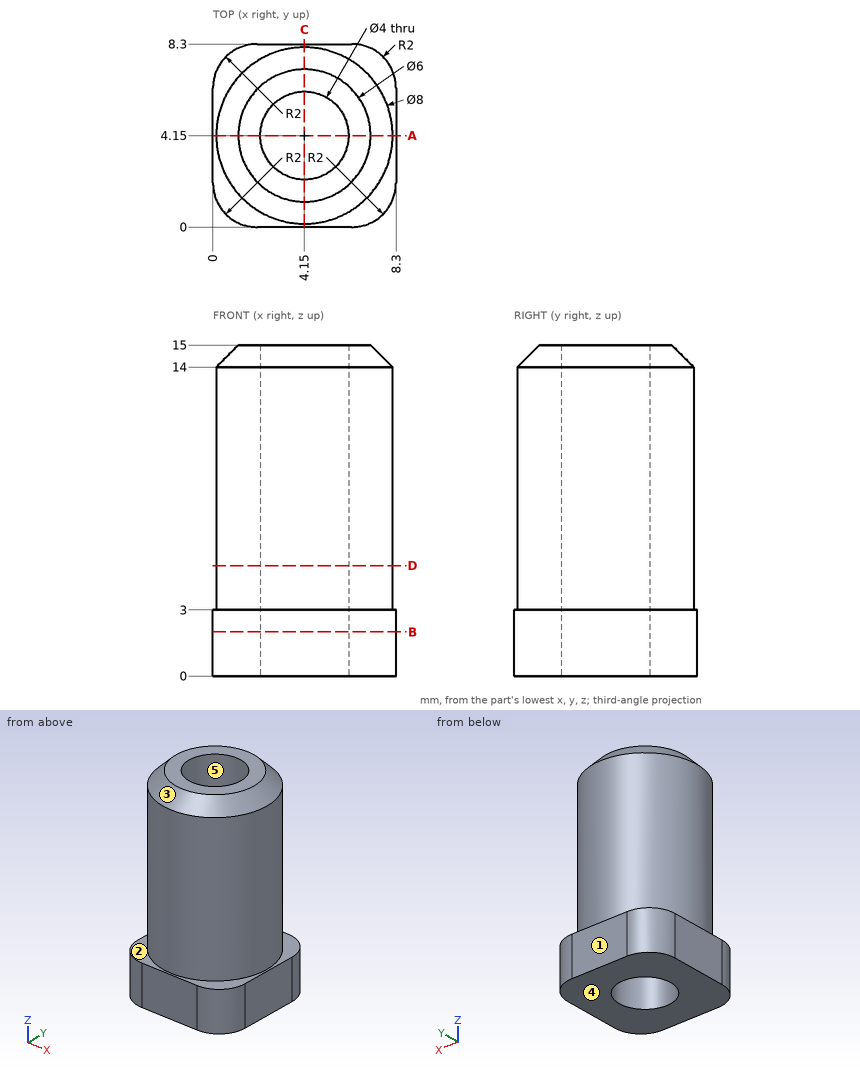
Could you check a few things on this drawing? It's one solid part, dimensions in mm from its lowest x, y, z. A direction names the side the tool comes from. Give positions to 0.01 mm unless a question says otherwise; leave off trailing zeros. Order: outer loops, then holes, each group sorted by start corner. A loop starts at its lowest first (then second) coordinate and runs counter-clockwise, first axis right, second up. Notation, with made-up numbers: (-13.75, 85.25) - (7.25, 85.25) arc R29 cw to (7.25, 113.25) - close; hole circle Ø10 at (5, 39.25). An arc over 180 degrees is marked (long way). Answer as a JSON object with one key per item and string values. Group by question number.
Item 1: For P1, Ø1.5, axis at x = 6.5, z = 11, coming from the +Y side, with a flat end and sliding along its axis, tell me the tip position at first contact or that it passes through.
Item 2: If we section it at D-D on z = 5: Please give me the cut outline in (x, y).
Item 3: If we mould it in two halves opening along X, with no side actions, what happens to the marked faces 3, 4 and 5? For each: pulls with the +X half, pulls with the -X half, needs draft (parallel to the pull), parting line crosses it, or undercut.
Item 4: If we section it at A-A on y = 4.15: Please give me the cut outline in (x, z).
Item 5: Please list where these lines run through material, in increasing order: probe 1 along Y at (x, z) = (4.15, 5); probe 2 along X at (y, z) = (4, 7.25); probe 3 along X at (y, z) = (4.75, 1.75).
Item 6: Which directions (+Z, -Z, +X, -X, +Y, -Y) give clear straight access to the entire face, cutting with the end or side of a thin tool? Please do the marked faces 1 and 2.
Item 7: If we section it at B-B on z = 2: Please give me the cut outline in (x, y), and give its area (3 significant figures).
Result set:
{
 "1": {"P1": "y = 7.82"},
 "2": {"outline": "circle Ø8 at (4.15, 4.15); hole circle Ø4 at (4.15, 4.15)"},
 "3": {"face 3": "parting line crosses it", "face 4": "needs draft", "face 5": "undercut"},
 "4": {"outline": "(0, 0) - (2.15, 0) - (2.15, 15) - (1.15, 15) - (0.15, 14) - (0.15, 3) - (0, 3) - close; (6.15, 0) - (8.3, 0) - (8.3, 3) - (8.15, 3) - (8.15, 14) - (7.15, 15) - (6.15, 15) - close"},
 "5": {"probe 1": "0.15 to 2.15, 6.15 to 8.15", "probe 2": "0.15 to 2.16, 6.14 to 8.15", "probe 3": "0 to 2.24, 6.06 to 8.3"},
 "6": {"face 1": "+Z, -Z, +X, -X, +Y", "face 2": "+Z"},
 "7": {"outline": "(0, 2) arc R2 ccw to (2, 0) - (6.3, 0) arc R2 ccw to (8.3, 2) - (8.3, 6.3) arc R2 ccw to (6.3, 8.3) - (2, 8.3) arc R2 ccw to (0, 6.3) - close; hole circle Ø4 at (4.15, 4.15)", "area": "52.9 mm²"}
}
